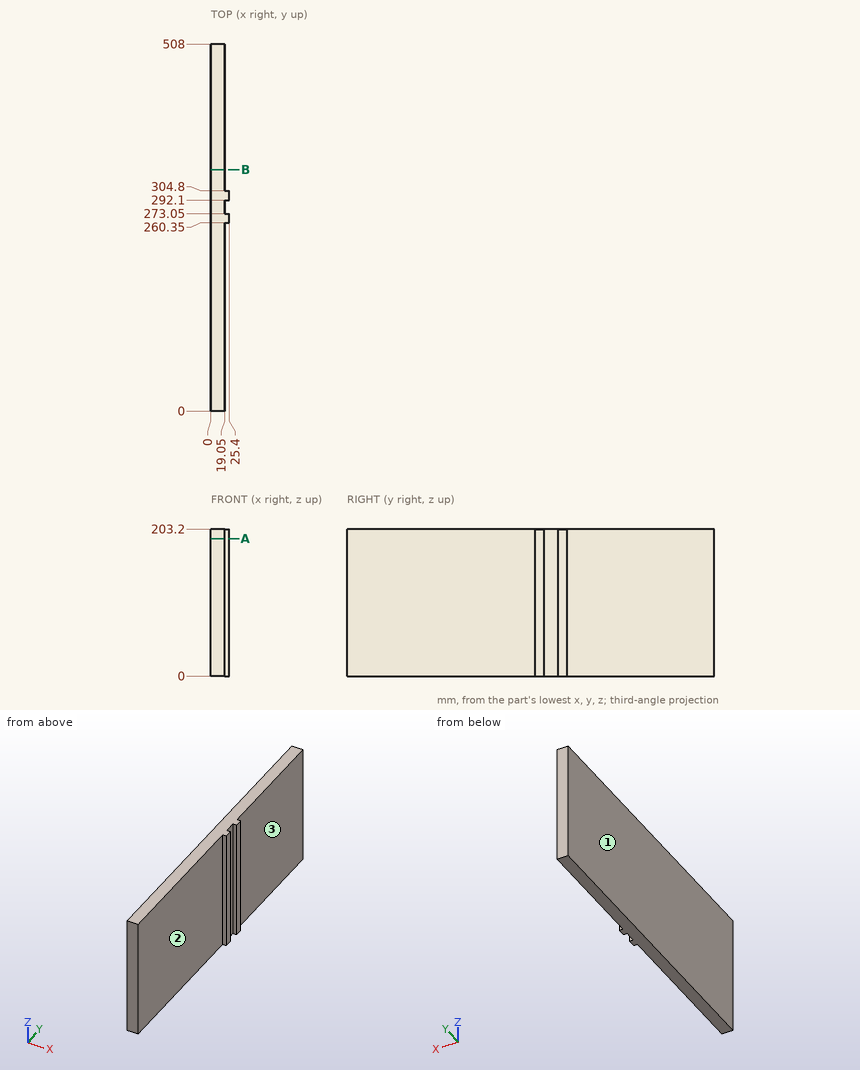
Part print with two shaded views. Sizes in mm from the minimum x, y, z corner. A direction names the side the tool comes from. Coordinates: 2 decimals unless noted, no trailing zeros. Write each loop counter-clockwise with the first axis right and the second up, starting at its lowest first coordinate (ties: lowest second). Pieces come first, ordered by that corner, then holes. Notation, with made-up numbers: M -9.5,-2 L 4.5,-2 A25 ccw 4.5,18 Z; hole C -13,-29 d10. An arc over 180 degrees is marked long. Return JSON: item names as keys, results as strings.
Item 1: Slice it at B-B, the plane y = 334. Write the cut outline in (x, z).
Findings below:
{"outline": "M 0,0 L 19.05,0 L 19.05,203.2 L 0,203.2 Z"}
Item 2: Slice it at A-A, the plane z = 190. Write the cut outline in (x, y), and give its area (3 significant figures).
Findings below:
{"outline": "M 0,0 L 19.05,0 L 19.05,260.35 L 25.4,260.35 L 25.4,273.05 L 19.05,273.05 L 19.05,292.1 L 25.4,292.1 L 25.4,304.8 L 19.05,304.8 L 19.05,508 L 0,508 Z", "area": "9,840 mm2"}
Item 3: Probe line 1 (Y direction, x = 24.25, z = 32); line 2 (X direction, y = 317, z = 121). List the from-to ranges inside material, lowest first. Write a range as from..to.
Findings below:
{"line 1": "y = 260.35..273.05, 292.1..304.8", "line 2": "x = 0..19.05"}
Item 4: Which spindle directions (+Z, -Z, +X, -X, +Y, -Y) get a long thin tool onto all of the face, cutting with end or side? Do the marked faces 1, 2 and 3. Say none if no direction does.
Findings below:
{"face 1": "+Z, -Z, -X, +Y, -Y", "face 2": "+Z, -Z, +X, -Y", "face 3": "+Z, -Z, +X, +Y"}
Item 5: Drop flat-ended pins along their axis: pin 1 Ø7 at (x, z) = (23, 147.5) entering from -Y; pin 2 Ø3 at (x, z) = (21, 87) entering from +Y; pin 3 Ø3 at (x, y) = (21.5, 386.5) entering from -Z; pin 4 Ø3 at (y, z) = (110.5, 179) entering from +X. Give the stop position or say it passes through.
Findings below:
{"pin 1": "stops at y = 260.35", "pin 2": "stops at y = 304.8", "pin 3": "passes through", "pin 4": "stops at x = 19.05"}
